For this review, take the finished solid that the model builds, in its own axes (mm). A direction names the side the tool comes from. Coordinates: 2 decimals unless noted, no trailing zeros. Write each loop counter-clockwise with the first axis right and the second up, starting at its lowest first coordinate (ties: lowest second). Pieces come first, ordered by that corner, then holes.
1) We need section A-A on x = 43.18. Write out the cut boundary in (y, z), then the cut area to 3 significant figures.
2) We need section C-C on x = -61. Write out the cut boundary in (y, z).
3) Insertion check: P1, Ø3, axis at x = -50.5, y = 9, coming from the +Z side; P2, Ø4, axis at x = -74, z = -3, coming from the +Y side; P3, Ø2, axis at y = 12, z = -3.5, coming from the -X side (3 decimals). Each pin has a flat end and moves straight along its axis. Give the tip position at first contact, or say it passes through.
4) For faces 4 (the face through (-77, 5, -37.592)), 5 (the face through (-77, 8.509, -29)), 6 (the face through (-77, 5, 1.778)), list the 3-axis set-ups (+Z, -Z, +X, -X, +Y, -Y) from which the entire face can be reached by the end or side of a thin tool; tool diameter is ignored.
5) We need section B-B on x = -34. Write out the cut boundary in (y, z).
6) To check wall thickness, follow line 1 along Z through (x, y) = (43.18, 14.75); line 2 along X through (y, z) = (2.25, 14) (3 decimals); line 3 along Z through (x, y) = (51, 3.5). State the ranges of each line that lie inside material, in increasing order.
7) Mouldability with a two-part tool opening along Z and no side actions: class faces 1 (the face through (-77, 5, 46.736)), 2 (the face through (-77, 5, -15.113)), 3 (the face through (-1, 0, 2)) as pulls with the +Z half, pulls with the -Z half, needs draft (parallel to the pull), parting line crosses it, or undercut.
from build123d import *

# Parameters (mm, degrees)
SKETCH1_W             = 167.64
SKETCH1_H             = 106.68
SKETCH1_W_2           = 99.06
SKETCH1_H_2           = 6.35
BOSS_EXTRUDE1_DEPTH   = 1.651
SKETCH2_W             = 135.255
SKETCH2_H             = 93.98
BOSS_EXTRUDE2_DEPTH   = 13.97
F_4_CLEARANCE_HOLE1_D = 3.175
SKETCH6_W             = 13.97
SKETCH6_H             = 16.891
BOSS_EXTRUDE3_DEPTH   = 6.858
SKETCH7_W             = 2.54
SKETCH7_H             = 12.7
CUT_EXTRUDE5_DEPTH    = 2.54
LPATTERN1_COUNT       = 18
LPATTERN1_PITCH       = 5.08
SKETCH8_R             = 26.9875
SKETCH8_R_2           = 12.7
CUT_EXTRUDE6_DEPTH    = 2.54


with BuildPart() as part:
    # Sketch1 → Boss-Extrude1 (new body)
    with BuildSketch(Plane(origin=(0, 0, 0), x_dir=(1, 0, 0), z_dir=(0, 1, 0))):
        Rectangle(SKETCH1_W, SKETCH1_H)
        with Locations((10.71, -56.515)):
            Rectangle(SKETCH1_W_2, SKETCH1_H_2)
    extrude(amount=BOSS_EXTRUDE1_DEPTH)

    # Sketch2 → Boss-Extrude2 (add)
    with BuildSketch(Plane(origin=(0, 1.651, 0), x_dir=(1, 0, 0), z_dir=(0, 1, 0))):
        with Locations((16.1925, 6.35)):
            Rectangle(SKETCH2_W, SKETCH2_H)
    extrude(amount=BOSS_EXTRUDE2_DEPTH)

    # #4 Clearance Hole1 (through all)
    with Locations(Plane(origin=(-78.9305, 1.651, -48.1965), x_dir=(0, 0, 1), z_dir=(0, 1, 0))):
        with Locations((0, 0), (98.3488, 2.286)):
            Hole(F_4_CLEARANCE_HOLE1_D / 2)

    # Sketch6 → Boss-Extrude3 (add)
    with BuildSketch(Plane(origin=(0, 1.651, 0), x_dir=(1, 0, 0), z_dir=(0, 1, 0))):
        with Locations((-76.835, 29.1465)):
            Rectangle(SKETCH6_W, SKETCH6_H)
        with Locations((-76.835, 6.6675)):
            Rectangle(SKETCH6_W, SKETCH6_H)
        with Locations((-76.835, -15.8115)):
            Rectangle(SKETCH6_W, SKETCH6_H)
        with Locations((-76.835, -38.2905)):
            Rectangle(SKETCH6_W, SKETCH6_H)
    extrude(amount=BOSS_EXTRUDE3_DEPTH)

    # Sketch7 → Cut-Extrude5 (cut)
    with BuildSketch(Plane.ZY.offset(51.435)):
        with Locations((36.83, 8.636)):
            Rectangle(SKETCH7_W, SKETCH7_H)
    cut_extrude5 = extrude(amount=-CUT_EXTRUDE5_DEPTH, mode=Mode.SUBTRACT)

    # LPattern1: Cut-Extrude5 ×18
    with Locations(*[(0, 0, -i * LPATTERN1_PITCH) for i in range(1, LPATTERN1_COUNT)]):
        add(cut_extrude5, mode=Mode.SUBTRACT)

    # Sketch8 → Cut-Extrude6 (cut)
    with BuildSketch(Plane(origin=(0, 15.621, 0), x_dir=(1, 0, 0), z_dir=(0, 1, 0))):
        with Locations((43.18, 12.7)):
            Circle(SKETCH8_R)
        with Locations((43.18, 12.7)):
            Circle(SKETCH8_R_2, mode=Mode.SUBTRACT)
    extrude(amount=-CUT_EXTRUDE6_DEPTH, mode=Mode.SUBTRACT)


solid = part.part
Result:
1. outline: (0, -53.34) - (15.62, -53.34) - (15.62, -39.69) - (13.08, -39.69) - (13.08, -25.4) - (15.62, -25.4) - (15.62, 0) - (13.08, 0) - (13.08, 14.29) - (15.62, 14.29) - (15.62, 40.64) - (1.65, 40.64) - (1.65, 59.69) - (0, 59.69) - close
1. area: 1,430 mm2
2. outline: (0, -53.34) - (1.65, -53.34) - (1.65, 53.34) - (0, 53.34) - close
3. P1: stops at z = 40.64
3. P2: stops at y = 8.51
3. P3: stops at x = -51.435
4. face 4: -Z, -X, +Y
4. face 5: +Z, -Z, -X, +Y
4. face 6: -X, +Y
5. outline: (0, -53.34) - (15.62, -53.34) - (15.62, 40.64) - (1.65, 40.64) - (1.65, 59.69) - (0, 59.69) - close
6. line 1: z = -53.34 to -39.69, -25.4 to 0, 14.29 to 40.64
6. line 2: x = -83.82 to -69.85, -51.435 to 83.82
6. line 3: z = -53.34 to 40.64
7. face 1: pulls with the +Z half
7. face 2: undercut
7. face 3: needs draft
